Geometry: final body of the model. Coordinates: model frame, mm. A direction names the side the tool comes from. Give positions to 0.01 mm unless a question says otherwise; leave off trailing zeros. Write each loop counter-clockwise with the first axis right and the second up, starting at its lowest first coordinate (ties: lowest second). Pieces come first, ordered by that corner, then holes. Notation, with made-up numbers: M -13,84 L 1,84 A18 cw 1,109 Z; hole C 2.25,-10 d5. An arc over 180 degrees is marked long. Use a Markdown table: item, result. Add a question column.
1) Pin query (flat end, axial travel): pin 1 (2 mm diameter, centred on x = 1.5, z = -4.5, fed in from +Y); pin 2 (0.8 mm diameter, centred on x = 0, y = 0, fed in from +Z); pin 3 (0.7 mm diameter, centred on x = -0.5, z = -1, fed in from -Y). Return the tip coordinate at first contact, or that it passes through.
2) Set-up query: faces 1 (the flat face through (-1.088, -0.616, -0.986)), 2 (the cylindrical face through (-0.54, -2.44, -1.33)). Return all of +Z, -Z, +X, -X, +Y, -Y with unobstructed straight access to the full face (end or side cutting, diameter ignored); none if empty.
3) Section C-C on z = -3.25. Return the cut outline in (x, y).
4) Section B-B on z = -1.9. Return the cut outline in (x, y).
5) Section A-A on x = 0. Return the cut outline in (y, z).
6) Draft query along X for faces 3 (the flat face through (-1.08, 0.63, -0.99)), 4 (the flat face through (1.1, -1.1, 0)), 5 (the conical face through (0.57, -0.18, -4.6)). Return one class per face: +X half, -X half, draft (parallel to the pull), parting line (faces both ways), or undercut.
7) Line query: line 1 (X direction, y = -0.65, z = -0.8); line 2 (X direction, y = -0.7, z = -0.6); line 3 (Z direction, x = -0.5, y = -0.35). Output: solid intervals per line, ascending.
```python
from build123d import *

# Parameters (mm, degrees)
SKETCH1_R           = 2.5
BOSS_EXTRUDE1_DEPTH = 5
CUT_EXTRUDE1_DEPTH  = 2


with BuildPart() as part:
    # Sketch1 → Boss-Extrude1 (new body)
    with BuildSketch(Plane.XY):
        Circle(SKETCH1_R)
    extrude(amount=-BOSS_EXTRUDE1_DEPTH)

    # Sketch2 → Cut-Extrude1 (cut)
    with BuildSketch(Plane.XY):
        Polygon((1.443375673, 0), (0.721687836, 1.25), (-0.721687836, 1.25), (-1.443375673, 0), (-0.721687836, -1.25), (0.721687836, -1.25), align=None)
    extrude(amount=-CUT_EXTRUDE1_DEPTH, mode=Mode.SUBTRACT)

    # Sketch3 → Chamfer 2 (revolve, cut)
    with BuildSketch(Plane(origin=(0, 0, 0), x_dir=(0, 0, -1), z_dir=(1, 0, 0)), mode=Mode.PRIVATE) as chamfer_2_sk:
        Polygon((5, 2.5), (5, 0.2), (2.7, 2.5), align=None)
    revolve(chamfer_2_sk.sketch.rotate(Axis((0, 0, 0), (0, 0, -1)), 90), axis=Axis((0, 0, 0), (0, 0, -1)), mode=Mode.SUBTRACT)


solid = part.part
```
Found:
| question | item | result |
|---|---|---|
| 1 | pin 1 | y = 1.21 |
| 1 | pin 2 | z = -2 |
| 1 | pin 3 | y = -2.5 |
| 2 | face 1 | +Z |
| 2 | face 2 | +Z, -Z |
| 3 | outline | C 0,0 d3.9 |
| 4 | outline | C 0,0 d5; hole M -1.44,0 L -0.72,-1.25 L 0.72,-1.25 L 1.44,0 L 0.72,1.25 L -0.72,1.25 Z |
| 5 | outline | M -2.5,-2.7 L -0.2,-5 L 0.2,-5 L 2.5,-2.7 L 2.5,0 L 1.25,0 L 1.25,-2 L -1.25,-2 L -1.25,0 L -2.5,0 Z |
| 6 | face 3 | undercut |
| 6 | face 4 | draft |
| 6 | face 5 | parting line |
| 7 | line 1 | -2.41 to -1.07, 1.07 to 2.41 |
| 7 | line 2 | -2.4 to -1.04, 1.04 to 2.4 |
| 7 | line 3 | -4.59 to -2 |
